Design review of the part shown in the three views and the two pictorial views. Dimensions are in mm from the part's minimum x, y and z. A direction names the side the tool comes from. Coordinates: 2 decimals unless noted, no trailing zeros. Write each loop counter-clockwise with the first axis right and the second up, starting at its lowest first coordinate (ties: lowest second). Pieces come first, ordered by that corner, then holes.
Q1. Take a section at A-A, the plane y = 24.5. Write out the cut boundary in (x, z), plus the area to 3 significant figures.
Q2. For L1, parallel to Z at x = 6.5, y = 14; L2, parallel to Y at x = 25, z = 6; L3, parallel to X at y = 45, z = 9.5, list the stretches that pass through material, from the lowest coordinate up.
Q3. Take a section at C-C, the plane z = 5. Write out the cut boundary in (x, y), plus the area to 3 significant figures.
Q4. For the marked faces 1 and 2, list the 3-axis set-ups (+Z, -Z, +X, -X, +Y, -Y) from which the entire face can be reached by the end or side of a thin tool; tool diameter is ignored.
Q5. For pin 1 Ø3 at (x, z) = (17, 23) entering from +Y; pin 2 Ø8 at (x, z) = (5, 44) entering from -Y; pin 3 Ø3 at (x, z) = (26.5, 47.5) entering from +Y, all flat-tipped, find the tip position at first contact; note any pin that passes through.
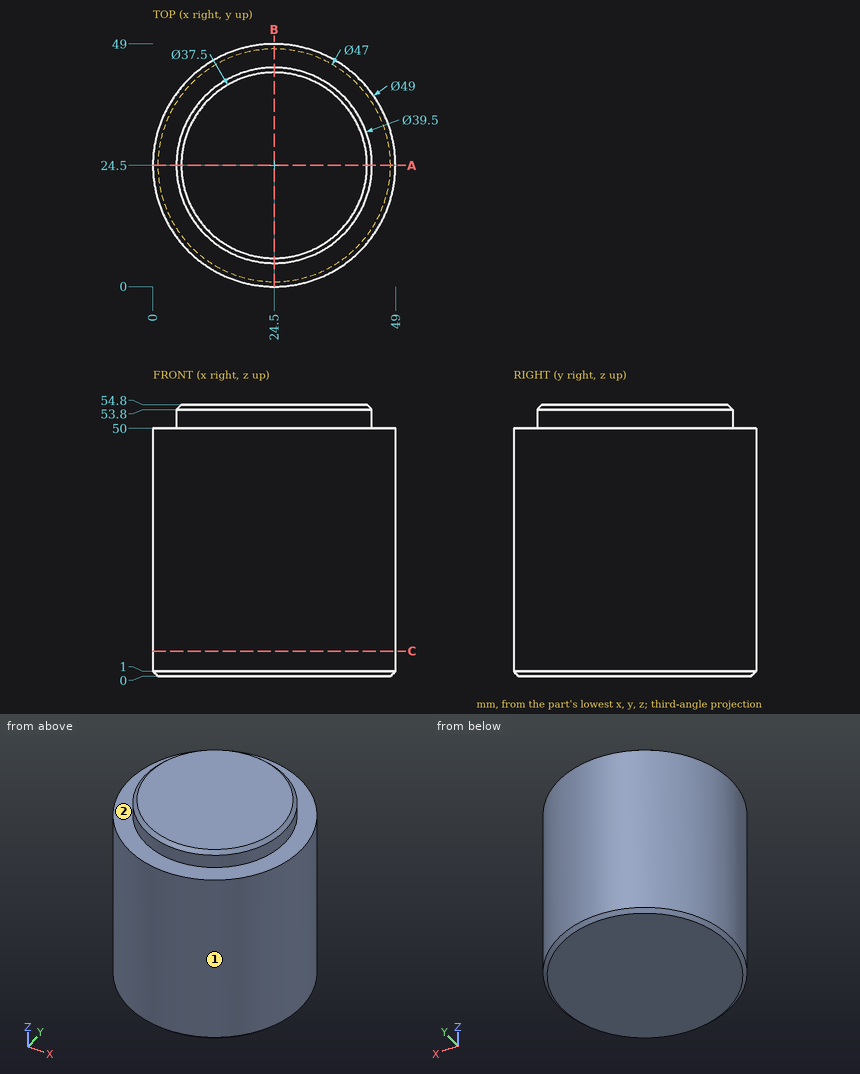
Responses:
1. outline: (0, 1) - (1, 0) - (48, 0) - (49, 1) - (49, 50) - (44.25, 50) - (44.25, 53.8) - (43.25, 54.8) - (5.75, 54.8) - (4.75, 53.8) - (4.75, 50) - (0, 50) - close
1. area: 2,640 mm2
2. L1: z = 0 to 50
2. L2: y = 0.01 to 48.99
2. L3: x = 11.08 to 37.92
3. outline: circle Ø49 at (24.5, 24.5)
3. area: 1,890 mm2
4. face 1: +Z, -Z
4. face 2: +Z
5. pin 1: stops at y = 48.25
5. pin 2: stops at y = 5.53
5. pin 3: stops at y = 48.99
